Here's how the part is built. I have some questions about the finished solid (model axes, mm). Face numbers are marked on the shaded views. Coordinates: 2 decimals unless noted, no trailing zeros. Write each loop counter-clockwise with the first axis right and the second up, starting at its lowest first coordinate (ties: lowest second). Pieces come first, ordered by that corner, then holes.
(1) For pin 1 Ø1.8 at (x, z) = (-211, -47.5) entering from +Y; pin 2 Ø3 at (x, z) = (-210.5, 66) entering from +Y; pin 3 Ø3 at (x, y) = (-210.5, 9.5) entering from -Z, each with a flat end and sliding along its axis, tell me the tip position at first contact or that it passes through.
(2) Imagine slicing it at C-C, the plane z = 48. List the corners of the cut face in (x, y) for me.
(3) Imagine slicing it at B-B, the plane y = 4. List the corners of the cut face in (x, z) for me.
(4) Imagine slicing it at A-A, the plane x = -212.15. List the corners of the cut face in (y, z) for me, plus the area to 3 significant figures.
(5) Please list where these lines run through material, in increasing order: probe 1 along Y at (x, z) = (-207.8, 8); probe 2 along Z at (x, y) = (-210.15, -25).
(6) Thinking about a two-plate mould opening in X: for the marked faces 1 and 2, which applies, released by +X, released by -X, zero draft, split by the parting line, or undercut?
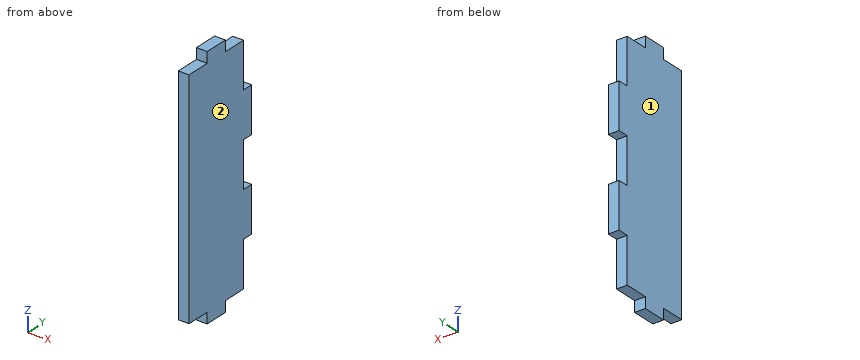
```python
from build123d import *

# Parameters (mm, degrees)
SKETCH1_W               = 415
SKETCH1_H               = 126.5
BOSS_EXTRUDE1_DEPTH     = 6
SKETCH2_W               = 6
SKETCH2_H               = 25.3
BOSS_EXTRUDE2_DEPTH     = 40
SKETCH1_2_W             = 415
SKETCH1_2_H             = 126.5
CUT_EXTRUDE1_DEPTH      = 7
CUT_EXTRUDE1_DEPTH_BACK = 35
SKETCH2_4_W             = 6
SKETCH2_4_H             = 25.3
BOSS_EXTRUDE3_DEPTH     = 6
SKETCH6_W               = 6
SKETCH6_H               = 13.333333334
BOSS_EXTRUDE5_DEPTH     = 6


with BuildPart() as part:
    # Sketch1 → Boss-Extrude1 (new body)
    with BuildSketch(Plane(origin=(0, 0, 0), x_dir=(1, 0, 0), z_dir=(0, 1, 0))):
        Rectangle(SKETCH1_W, SKETCH1_H)
    extrude(amount=BOSS_EXTRUDE1_DEPTH)

    # Sketch2 → Boss-Extrude2 (add)
    with BuildSketch(Plane(origin=(0, 6, 0), x_dir=(1, 0, 0), z_dir=(0, 1, 0))):
        with Locations((-210.5, 50.6)):
            Rectangle(SKETCH2_W, SKETCH2_H)
        with Locations((-210.5, 25.3)):
            Rectangle(SKETCH2_W, SKETCH2_H)
        with Locations((-210.5, 0)):
            Rectangle(SKETCH2_W, SKETCH2_H)
        with Locations((-210.5, -25.3)):
            Rectangle(SKETCH2_W, SKETCH2_H)
        with Locations((-210.5, -50.6)):
            Rectangle(SKETCH2_W, SKETCH2_H)
    extrude(amount=-BOSS_EXTRUDE2_DEPTH)

    # Sketch1<2> → Cut-Extrude1 (cut, two sides)
    with BuildSketch(Plane(origin=(0, 0, 0), x_dir=(1, 0, 0), z_dir=(0, 1, 0))) as cut_extrude1_sk:
        Rectangle(SKETCH1_2_W, SKETCH1_2_H)
    extrude(amount=CUT_EXTRUDE1_DEPTH, mode=Mode.SUBTRACT)
    extrude(cut_extrude1_sk.sketch, amount=-CUT_EXTRUDE1_DEPTH_BACK, mode=Mode.SUBTRACT)

    # Sketch2<4> → Boss-Extrude3 (add)
    with BuildSketch(Plane(origin=(0, 6, 0), x_dir=(1, 0, 0), z_dir=(0, 1, 0))):
        with Locations((-210.5, -25.3)):
            Rectangle(SKETCH2_4_W, SKETCH2_4_H)
        with Locations((-210.5, 25.3)):
            Rectangle(SKETCH2_4_W, SKETCH2_4_H)
    extrude(amount=BOSS_EXTRUDE3_DEPTH)

    # Sketch6 → Boss-Extrude5 (add)
    with BuildSketch(Plane.XY.offset(63.25)):
        with Locations((-210.5, -14)):
            Rectangle(SKETCH6_W, SKETCH6_H)
    boss_extrude5 = extrude(amount=BOSS_EXTRUDE5_DEPTH)

    # Mirror4: Boss-Extrude5 across plane
    add(boss_extrude5.mirror(Plane.XY))


solid = part.part
```
Recorded:
1. pin 1: stops at y = 6
1. pin 2: stops at y = -7.33
1. pin 3: stops at z = -37.95
2. outline: (-213.5, -34) - (-207.5, -34) - (-207.5, 6) - (-213.5, 6) - close
3. outline: (-213.5, -63.25) - (-207.5, -63.25) - (-207.5, 63.25) - (-213.5, 63.25) - close
4. outline: (-34, -63.25) - (-20.67, -63.25) - (-20.67, -69.25) - (-7.33, -69.25) - (-7.33, -63.25) - (6, -63.25) - (6, -37.95) - (12, -37.95) - (12, -12.65) - (6, -12.65) - (6, 12.65) - (12, 12.65) - (12, 37.95) - (6, 37.95) - (6, 63.25) - (-7.33, 63.25) - (-7.33, 69.25) - (-20.67, 69.25) - (-20.67, 63.25) - (-34, 63.25) - close
4. area: 5,520 mm2
5. probe 1: y = -34 to 6
5. probe 2: z = -63.25 to 63.25
6. face 1: released by -X
6. face 2: released by +X
